from build123d import *

# Parameters (mm, degrees)
SKETCH_4_R          = 33.5
EXTRUDE_1_DEPTH     = 26.5
SKETCH_5_R          = 3
CUT_EXTRUDE_1_DEPTH = 9
EXTRUDE_START       = 2.5
SKETCH_6_R          = 5.75
SKETCH_6_R_2        = 3
EXTRUDE_3_DEPTH     = 2.5


with BuildPart() as part:
    # 草图4 → 凸台-拉伸1 (new body)
    with BuildSketch(Plane(origin=(0, 0, 0), x_dir=(0, 0, -1), z_dir=(1, 0, 0))):
        Circle(SKETCH_4_R)
    extrude(amount=EXTRUDE_1_DEPTH)

    # 草图5 → 切除-拉伸1 (cut)
    with BuildSketch(Plane.ZY):
        Circle(SKETCH_5_R)
    extrude(amount=-CUT_EXTRUDE_1_DEPTH, mode=Mode.SUBTRACT)

    # 草图6 → 凸台-拉伸3 (add)
    with BuildSketch(Plane.ZY.offset(EXTRUDE_START)):
        with Locations(Location((0, 0, 0), (0, 0, 180))):
            Circle(SKETCH_6_R)
        Circle(SKETCH_6_R_2, mode=Mode.SUBTRACT)
    extrude(amount=-EXTRUDE_3_DEPTH)


solid = part.part
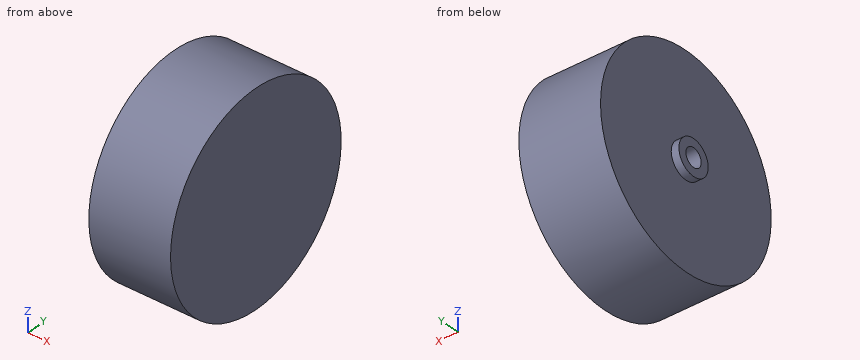
Can you work these out from the model? Positions are in its coordinate system, mm. Coordinates: 2 decimals unless noted, no trailing zeros. Write each loop counter-clockwise with the first axis right and the second up, starting at its lowest first coordinate (ties: lowest second). Pieces come first, ordered by that corner, then holes. Notation, with made-up numbers: (40.5, -31.5) -> (86.5, -31.5) arc R11 ccw to (86.5, -13.5) -> close; hole circle Ø10 at (78.25, 32). An arc over 180 degrees is marked (long way). Write each question's results on one line, items separated by ' | '. Start each with the question number.
Item 1: If we section it at A-A, the plane z = 0: Write out the boundary of the cut face in (x, y).
Item 2: If we section it at D-D, the plane x = 7.5: Write out the boundary of the cut face in (y, z), and give its area (3 significant figures).
Item 3: I'm going to push flat-ended pins straight in: P1, Ø6, axis at x = 21.5, y = 26, coming from the +Z side; P2, Ø10, axis at y = -8, z = -7.5, coming from the -X side; P3, Ø8, axis at y = 1, z = 6.5, coming from the -X side; P4, Ø2, axis at x = 17, z = 4, coming from the -Y side. Where does each tip first touch, or does it pass through?
Item 4: If we section it at C-C, the plane x = 12: Write out the boundary of the cut face in (y, z).
Item 5: Please list where these lines run through material, in increasing order: probe 1 along Y at (x, z) = (4, 0); probe 2 along X at (y, z) = (-14, -0.5); probe 3 along Z at (x, y) = (4, -20.5).
Answer block:
1) outline: (-2.5, -5.75) -> (0, -5.75) -> (0, -33.5) -> (26.5, -33.5) -> (26.5, 33.5) -> (0, 33.5) -> (0, 5.75) -> (-2.5, 5.75) -> (-2.5, 3) -> (9, 3) -> (9, -3) -> (-2.5, -3) -> close
2) outline: circle Ø67 at (0, 0); hole circle Ø6 at (0, 0) | area: 3,500 mm²
3) P1: z = 24.36 | P2: x = 0 | P3: x = -2.5 | P4: y = -33.37
4) outline: circle Ø67 at (0, 0)
5) probe 1: -33.5 to -3, 3 to 33.5 | probe 2: 0 to 26.5 | probe 3: -26.5 to 26.5
